Job drawing, mm, ordinate dimensions from the low corner. One solid piece. A direction names the side the tool comes from. Give positions to 0.01 mm unless a question says otherwise; leave off trailing zeros. Order: outer loops, then holes, each group sorted by start corner. A loop starts at its lowest first (then second) coordinate and runs counter-clockwise, first axis right, second up. Notation, with made-up numbers: (36, 23.5) -> (80, 23.5) arc R16 ccw to (80, 45.5) -> close; hole circle Ø2 at (-38.5, -35). An arc over 180 degrees is marked (long way). Write item = value, one per line. Start each with the question number.
(1) Saw through at A-A, the plane x = 6.5. List the corners of the cut face in (y, z).
(2) Probe line 1 along Y through (x, z) = (5, 6.5); line 2 along Y through (x, z) = (5, 8); line 3 along X through (y, z) = (43.5, 5.25). List the from-to ranges inside material, lowest first. Write a range as from..to.
(3) Two-plate mould, pull along X, no slides. Class the marked faces 4, 5 and 6: pulls with the +X half, pulls with the -X half, needs draft (parallel to the pull), parting line crosses it, or undercut.
(4) Flat gauge pins, fed straight in: pin 1 (1.2 mm diameter, centred on x = 6, z = 6, fed in from +Y); pin 2 (1.5 mm diameter, centred on x = 5, y = 20, fed in from -Z); pin 3 (1.5 mm diameter, centred on y = 14.5, z = 5.5, fed in from +X). Where does each tip first touch, or does it go through?
(5) Saw through at D-D, the plane y = 18.5. List the corners of the cut face in (x, z).
(6) Saw through at C-C, the plane z = 10. List the corners of the cut face in (x, y).
(7) Saw through at B-B, the plane y = 41.5. List the corners of the cut face in (x, z), then the cut area to 3 significant figures.
(8) Which spindle directions (+Z, -Z, +X, -X, +Y, -Y) get a long thin tool onto all of the face, cutting with end or side? Do the marked faces 1, 2 and 3. Say none if no direction does.
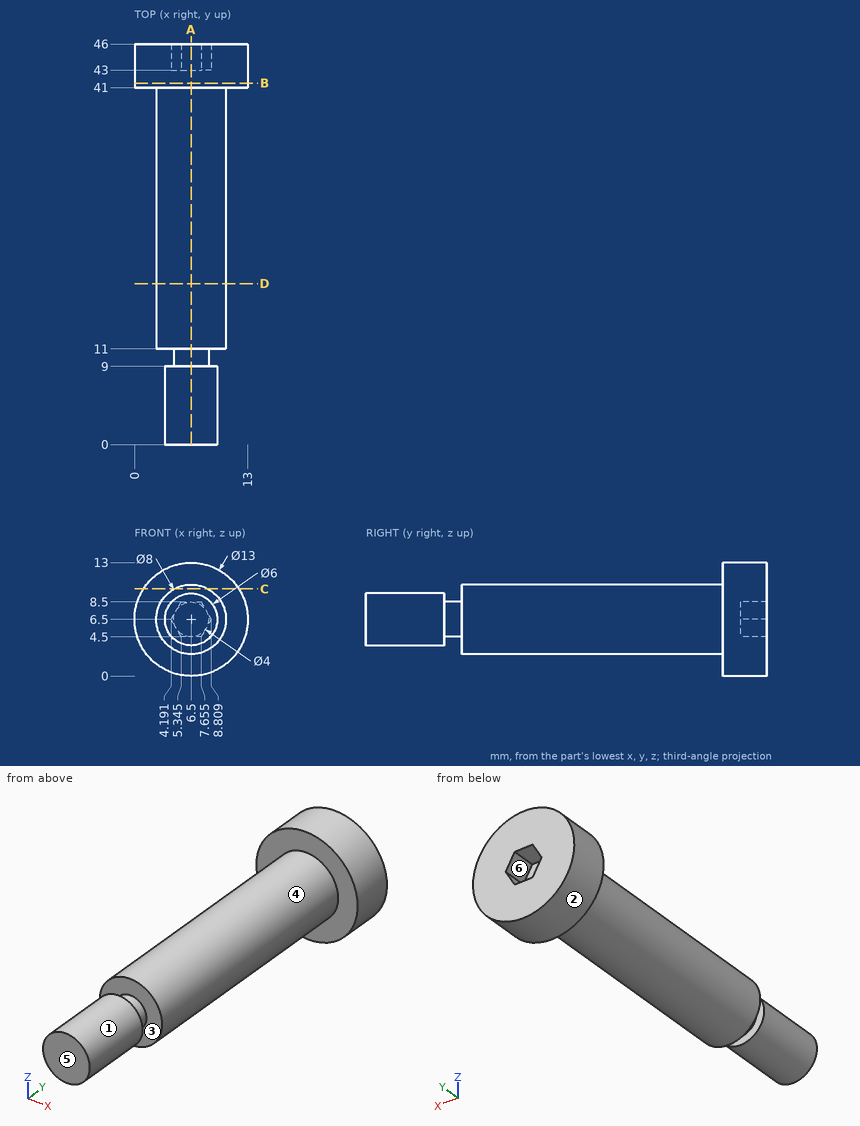
Results list:
q1.outline = (0, 3.5) -> (9, 3.5) -> (9, 4.5) -> (11, 4.5) -> (11, 2.5) -> (41, 2.5) -> (41, 0) -> (46, 0) -> (46, 4.5) -> (43, 4.5) -> (43, 8.5) -> (46, 8.5) -> (46, 13) -> (41, 13) -> (41, 10.5) -> (11, 10.5) -> (11, 8.5) -> (9, 8.5) -> (9, 9.5) -> (0, 9.5) -> close
q2.line_1 = 0..43
q2.line_2 = 0..9, 11..46
q2.line_3 = 0.12..4.91, 8.09..12.88
q3.face_4 = parting line crosses it
q3.face_5 = needs draft
q3.face_6 = undercut
q4.pin_1 = 43
q4.pin_2 = 2.57
q4.pin_3 = 10.49
q5.outline = circle Ø8 at (6.5, 6.5)
q6.outline = (1.02, 41) -> (4.56, 41) -> (4.56, 11) -> (8.44, 11) -> (8.44, 41) -> (11.98, 41) -> (11.98, 46) -> (1.02, 46) -> close
q7.outline = circle Ø13 at (6.5, 6.5)
q7.area = 133 mm^2
q8.face_1 = -Y
q8.face_2 = +Y, -Y
q8.face_3 = none
